Could you check a few things on this drawing? It's one solid part, dimensions in mm from its lowest x, y, z. A direction names the side the tool comes from. Give positions to 0.01 mm unless a question says otherwise; leave off trailing zeros. Loops run counter-clockwise (first coordinate to the right, second up) from the corner with the lowest first, then second, coordinate; pieces in that order, holes last. Notation, with made-up numbers: M 32.5,75 L 59.5,75 A33 ccw 59.5,103 Z; hole C 30.25,26.25 d3. An arc over 180 degrees is marked long. One line per item, written item: value. Start each with the question number.
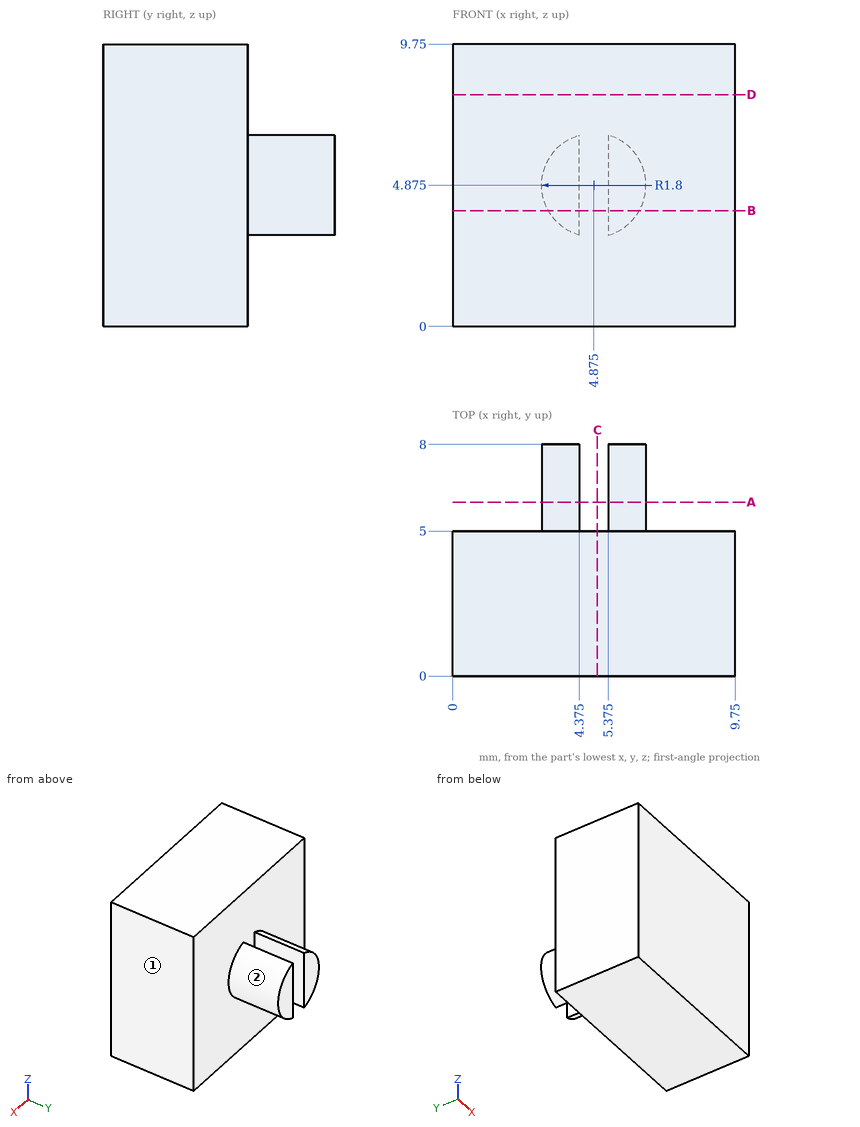
Q1. If we section it at D-D, the plane z = 8: Write out the boundary of the cut face in (x, y).
Q2. If we section it at A-A, the plane y = 6: Write out the boundary of the cut face in (x, z) (3 decimals), plus the area to 3 significant figures.
Q3. For P1, Ø1.5, axis at x = 8, z = 1.5, coming from the +Y side; P2, Ø2.5, axis at y = 7, z = 5.5, coming from the +X side (3 decimals), each with a flat end and sliding along its axis, tell me the tip position at first contact or that it passes through.
Q4. If we section it at C-C, the plane x = 5: Write out the boundary of the cut face in (y, z).
Q5. I need wall thicknesses on line 1 along Y through (x, z) = (4.25, 3); line 2 along X through (y, z) = (6.5, 6.5) (3 decimals); line 3 along Z through (x, y) = (6, 7.25). Which ranges of each line are inside material? Lowest first, please.
Q6. If we section it at B-B, the plane z = 4: Write out the boundary of the cut face in (x, y) (3 decimals), plus the area to 3 significant figures.
Q7. Which directions (+Z, -Z, +X, -X, +Y, -Y) give clear straight access to the entire face, cutting with the end or side of a thin tool? Please do the marked faces 1 and 2.
Response:
1. outline: M 0,0 L 9.75,0 L 9.75,5 L 0,5 Z
2. outline: M 4.375,3.146 L 4.375,6.604 A1.8 ccw Z; M 5.375,3.146 A1.8 ccw 5.375,6.604 Z
2. area: 6.63 mm^2
3. P1: y = 5
3. P2: x = 6.675
4. outline: M 0,0 L 5,0 L 5,9.75 L 0,9.75 Z
5. line 1: 0 to 5
5. line 2: 4.101 to 4.375, 5.375 to 5.649
5. line 3: 3.47 to 6.28
6. outline: M 0,0 L 9.75,0 L 9.75,5 L 6.448,5 L 6.448,8 L 5.375,8 L 5.375,5 L 4.375,5 L 4.375,8 L 3.302,8 L 3.302,5 L 0,5 Z
6. area: 55.2 mm^2
7. face 1: +Z, -Z, +X, +Y, -Y
7. face 2: +X, +Y
